Source: three-view drawing plus pictorial views. Frame: mm from the lowest corner of the part. Coordinates: 2 decimals unless noted, no trailing zeros. Order: outer loops, then holes, each group sorted by start corner. A loop starts at its lowest first (then second) coordinate and runs counter-clockwise, first axis right, second up. Notation, with made-up numbers: M 89.25,61.5 L 135.25,61.5 A14 cw 135.25,84.5 Z; hole C -40,33.5 d7. An arc over 180 degrees is marked long. Use CSV: the item, a comma, the result in double quotes. Start each with the question number.
Q1. Section query A-A, the plane y = 18.5. Output: boundary loops of the cut face in (x, z).
Q2. Section query B-B, the plane z = 25.5. Output: boundary loops of the cut face in (x, y), and give its area (3 significant figures).
Q3. First-contact query: P1, Ø12, axis at x = 252, z = 20, coming from the +Y side; P2, Ø4, axis at y = 24, z = 15.5, coming from the -X side. Flat tips, straight axial feed; report the tip coordinate or a pass-through.
Q4. Section query C-C, the plane x = 298. Output: boundary loops of the cut face in (y, z), and give its area (3 significant figures).
Q5. Ray query, probe 1 along X at (y, z) = (7, 16); probe 2 along Z at (x, y) = (128.5, 19); probe 3 along Y at (x, z) = (297, 20). Return the intervals inside material, ascending.
Q6. Section query D-D, the plane x = 225.5. Output: boundary loops of the cut face in (y, z).
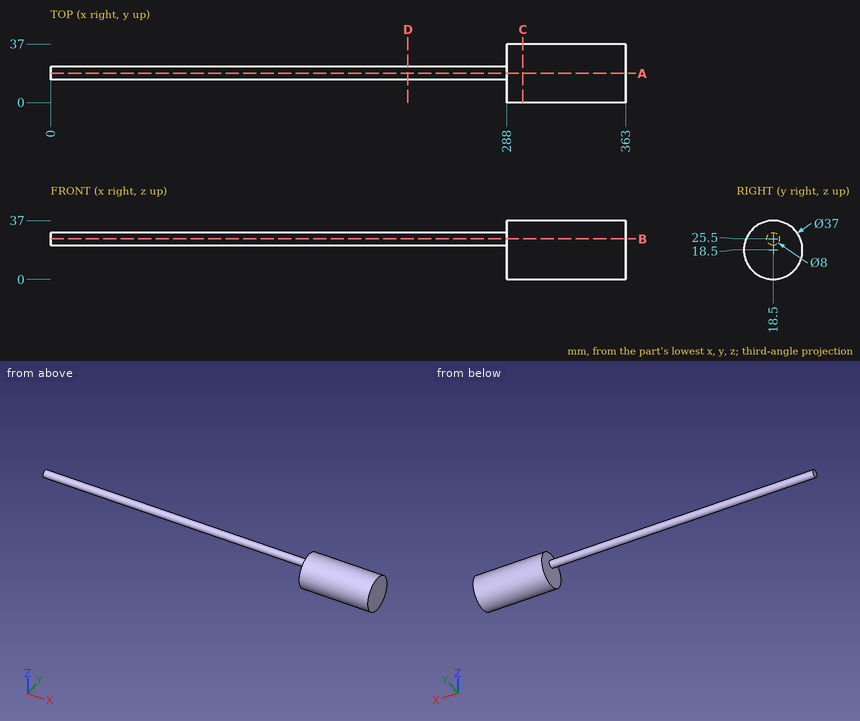
Responses:
1,outline,"M 0,21.5 L 288,21.5 L 288,0 L 363,0 L 363,37 L 288,37 L 288,29.5 L 0,29.5 Z"
2,outline,"M 0,14.5 L 288,14.5 L 288,1.38 L 363,1.38 L 363,35.62 L 288,35.62 L 288,22.5 L 0,22.5 Z"
2,area,"4,870 mm²"
3,P1,"stops at y = 22.5"
3,P2,"stops at x = 288"
4,outline,"C 18.5,18.5 d37"
4,area,"1,080 mm²"
5,probe 1,"x = 288 to 363"
5,probe 2,"z = 21.53 to 29.47"
5,probe 3,"y = 0.06 to 36.94"
6,outline,"C 18.5,25.5 d8"
